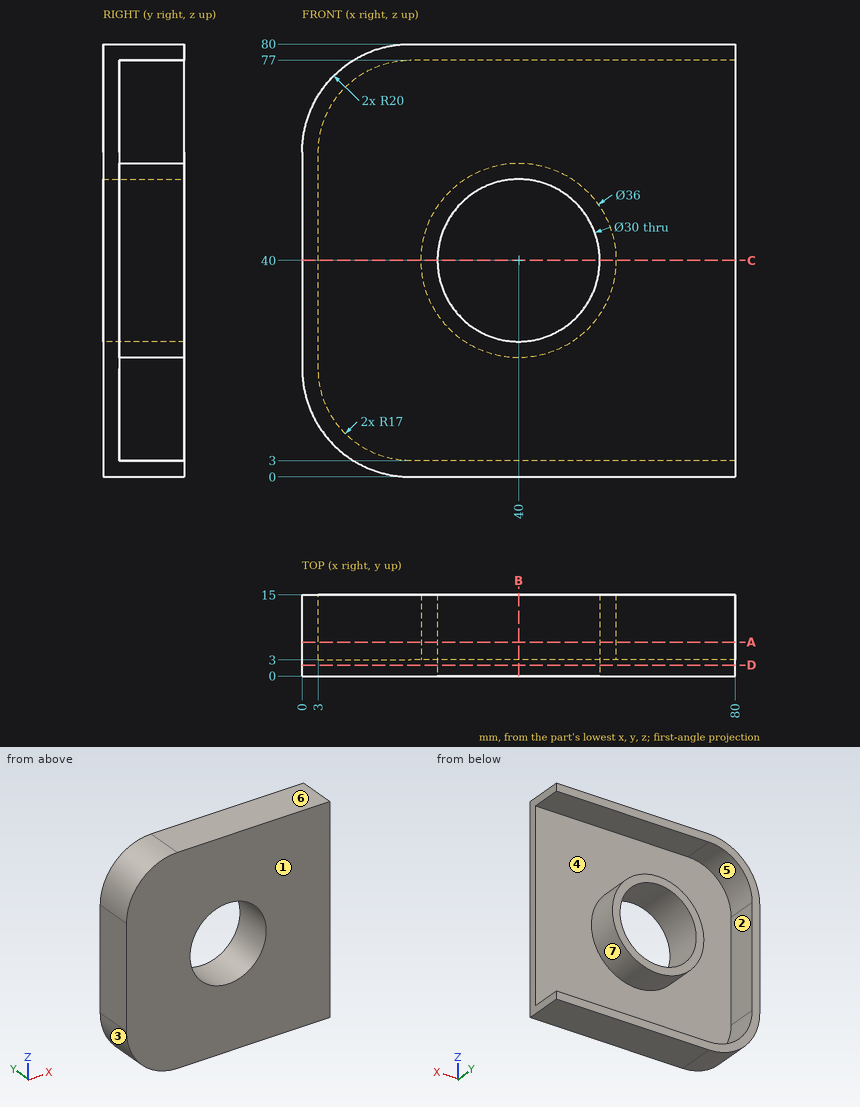
For this review, use the dimensioned drawing (mm, ordinates from the lowest corner) and the shaded views. A direction names the side the tool comes from. Coordinates: 2 decimals unless noted, no trailing zeros. Loops run counter-clockwise (first coordinate to the right, second up) from the corner with the lowest first, then second, coordinate; pieces in that order, holes last. Notation, with made-up numbers: (36.5, 8.5) -> (76.5, 8.5) arc R11 cw to (76.5, 18.5) -> close; hole circle Ø10 at (65, 86.25). An arc over 180 degrees is marked (long way). Use a Markdown table: item, result. Add a question column.
Item 1: Machinability: for the marked faces 5, 6 and 7, which of the approach directions +Z, -Z, +X, -X, +Y, -Y give a long, thin tool a straight path to every point of the face, cutting with its end or side? Answer none if there is none.
Item 2: Wall thickness on L1, parallel to X at y = 5, z = 40; L2, parallel to Z at x = 42, y = 7.75; L3, parallel to Z at x = 44, y = 11.5: over which ranges is each line inside the solid? List them lowest first. Write a range as from..to.
Item 3: The part is to be moulded in two halves that separate along Z. For the marked faces 1, 2, 3 and 4, say which applies: +Z half, -Z half, draft (parallel to the pull), parting line (faces both ways), or undercut.
Item 4: We need section B-B, the plane x = 40. Write out the cut boundary in (y, z).
Item 5: We need section A-A, the plane y = 6.25. Write out the cut boundary in (x, z).
Item 6: We need section D-D, the plane y = 2. Write out the cut boundary in (x, z).
Item 7: We need section C-C, the plane z = 40. Write out the cut boundary in (x, y).
Numbers:
| question | item | result |
|---|---|---|
| 1 | face 5 | +X, +Y |
| 1 | face 6 | +Z, +X, -X, +Y, -Y |
| 1 | face 7 | +Y |
| 2 | L1 | x = 0..3, 22..25, 55..58 |
| 2 | L2 | z = 0..3, 22.11..25.13, 54.87..57.89, 77..80 |
| 2 | L3 | z = 0..3, 22.45..25.54, 54.46..57.55, 77..80 |
| 3 | face 1 | draft |
| 3 | face 2 | undercut |
| 3 | face 3 | -Z half |
| 3 | face 4 | undercut |
| 4 | outline | (0, 0) -> (15, 0) -> (15, 3) -> (3, 3) -> (3, 22) -> (15, 22) -> (15, 25) -> (0, 25) -> close; (0, 55) -> (15, 55) -> (15, 58) -> (3, 58) -> (3, 77) -> (15, 77) -> (15, 80) -> (0, 80) -> close |
| 5 | outline | (0, 20) arc R20 ccw to (20, 0) -> (80, 0) -> (80, 3) -> (20, 3) arc R17 cw to (3, 20) -> (3, 60) arc R17 cw to (20, 77) -> (80, 77) -> (80, 80) -> (20, 80) arc R20 ccw to (0, 60) -> close; circle Ø36 at (40, 40); hole circle Ø30 at (40, 40) |
| 6 | outline | (0, 20) arc R20 ccw to (20, 0) -> (80, 0) -> (80, 80) -> (20, 80) arc R20 ccw to (0, 60) -> close; hole circle Ø30 at (40, 40) |
| 7 | outline | (0, 0) -> (25, 0) -> (25, 15) -> (22, 15) -> (22, 3) -> (3, 3) -> (3, 15) -> (0, 15) -> close; (55, 0) -> (80, 0) -> (80, 3) -> (58, 3) -> (58, 15) -> (55, 15) -> close |
